Source: CAD feature listing. Evaluate the final solid. Frame: model axes, mm. A direction names the side the tool comes from. Give positions to 0.01 mm unless a question says otherwise; leave off trailing zeros. Order: outer loops, then holes, each group sorted by start corner. A loop starts at its lowest first (then second) coordinate and runs counter-clockwise, first axis right, second up.
```python
from build123d import *

# Parameters (mm, degrees)
SKETCH1_W               = 41
SKETCH1_H               = 30
BOSS_EXTRUDE1_DEPTH     = 20.4
SHELL1_T                = 2
BOSS_EXTRUDE2_START     = -2
BOSS_EXTRUDE2_OUTLINE_W = 5
BOSS_EXTRUDE2_OUTLINE_H = 20.4
BOSS_EXTRUDE2_OUTLINE_R = 2.25
BOSS_EXTRUDE2_DEPTH     = 2
SKETCH3_W               = 5
SKETCH3_H               = 2
BOSS_EXTRUDE3_DEPTH     = 2
SKETCH4_W               = 5
SKETCH4_H               = 2
BOSS_EXTRUDE4_DEPTH     = 2
SKETCH5_W               = 5
SKETCH5_H               = 2
BOSS_EXTRUDE5_DEPTH     = 2
SKETCH6_W               = 5
SKETCH6_H               = 2
BOSS_EXTRUDE6_DEPTH     = 2
SKETCH7_W               = 5
SKETCH7_H               = 30
BOSS_EXTRUDE7_DEPTH     = 1
SKETCH9_R               = 4.146052681
CUT_EXTRUDE4_DEPTH      = 11
SKETCH10_W              = 55
SKETCH10_H              = 32
BOSS_EXTRUDE9_DEPTH     = 2
BOSS_EXTRUDE10_DEPTH    = 3
FILLET1_R               = 1
SKETCH18_W              = 26.995153054
SKETCH18_H              = 16.789310936
CUT_EXTRUDE5_DEPTH      = 10
SKETCH20_R              = 2.5
CUT_EXTRUDE7_DEPTH      = 10


# Read off the part's stored shape, not the designer's step: Boss-Extrude2
with BuildPart() as part:
    # Sketch1 → Boss-Extrude1 (new body)
    with BuildSketch(Plane(origin=(0, 0, 0), x_dir=(1, 0, 0), z_dir=(0, 1, 0))):
        with Locations((20.5, 15)):
            Rectangle(SKETCH1_W, SKETCH1_H)
    extrude(amount=BOSS_EXTRUDE1_DEPTH)

    # Shell1
    shell1_openings = [part.faces().sort_by_distance(p)[0] for p in [
        (20.5, 10.2, 0),
    ]]
    offset(amount=SHELL1_T, openings=shell1_openings, kind=Kind.INTERSECTION)

    # Boss-Extrude2 outline → Boss-Extrude2 (add)
    # profile 1 of 2: a face of its own
    with BuildSketch(Plane.XY.offset(BOSS_EXTRUDE2_START)):
        with Locations((-4.5, 10.2)):
            Rectangle(BOSS_EXTRUDE2_OUTLINE_W, BOSS_EXTRUDE2_OUTLINE_H)
        with Locations((-4.5, 5.5)):
            Circle(BOSS_EXTRUDE2_OUTLINE_R, mode=Mode.SUBTRACT)
        with Locations((-4.5, 14.9)):
            Circle(BOSS_EXTRUDE2_OUTLINE_R, mode=Mode.SUBTRACT)
    # profile 2 of 2: a face of its own
    with BuildSketch(Plane.XY.offset(BOSS_EXTRUDE2_START)):
        with Locations((45.5, 10.2)):
            Rectangle(BOSS_EXTRUDE2_OUTLINE_W, BOSS_EXTRUDE2_OUTLINE_H)
        with Locations((45.5, 5.5)):
            Circle(BOSS_EXTRUDE2_OUTLINE_R, mode=Mode.SUBTRACT)
        with Locations((45.5, 14.9)):
            Circle(BOSS_EXTRUDE2_OUTLINE_R, mode=Mode.SUBTRACT)
    extrude(amount=BOSS_EXTRUDE2_DEPTH)

    # Sketch3 → Boss-Extrude3 (add)
    with BuildSketch(Plane(origin=(0, 20.4, 0), x_dir=(1, 0, 0), z_dir=(0, 1, 0))):
        with Locations((-4.5, 1)):
            Rectangle(SKETCH3_W, SKETCH3_H)
    extrude(amount=BOSS_EXTRUDE3_DEPTH)

    # Sketch4 → Boss-Extrude4 (add)
    with BuildSketch(Plane.XZ):
        with Locations((-4.5, -1)):
            Rectangle(SKETCH4_W, SKETCH4_H)
    extrude(amount=BOSS_EXTRUDE4_DEPTH)

    # Sketch5 → Boss-Extrude5 (add)
    with BuildSketch(Plane(origin=(0, 20.4, 0), x_dir=(1, 0, 0), z_dir=(0, 1, 0))):
        with Locations((45.5, 1)):
            Rectangle(SKETCH5_W, SKETCH5_H)
    extrude(amount=BOSS_EXTRUDE5_DEPTH)

    # Sketch6 → Boss-Extrude6 (add)
    with BuildSketch(Plane.XZ):
        with Locations((45.5, -1)):
            Rectangle(SKETCH6_W, SKETCH6_H)
    extrude(amount=BOSS_EXTRUDE6_DEPTH)

    # Sketch7 → Boss-Extrude7 (add)
    with BuildSketch(Plane.XZ.offset(2)):
        Polygon((-7, -2), (-2, -2), (-2, -32), (43, -32), (43, -2), (48, -2), (48, 0), (-7, 0), align=None)
        with Locations((-4.5, -17)):
            Rectangle(SKETCH7_W, SKETCH7_H)
        with Locations((45.5, -17)):
            Rectangle(SKETCH7_W, SKETCH7_H)
    extrude(amount=BOSS_EXTRUDE7_DEPTH)

    # Sketch9 → Cut-Extrude4 (cut)
    with BuildSketch(Plane(origin=(0, 0, -2), x_dir=(-1, 0, 0), z_dir=(0, 0, -1))):
        with Locations((4.5, 5.5)):
            Circle(SKETCH9_R)
        with Locations((4.5, 14.9)):
            Circle(SKETCH9_R)
    cut_extrude4 = extrude(amount=CUT_EXTRUDE4_DEPTH, mode=Mode.SUBTRACT)

    # Mirror1: Cut-Extrude4 across plane
    add(cut_extrude4.mirror(Plane(origin=(20.5, 0, 0), x_dir=(0, 0, 1), z_dir=(1, 0, 0))), mode=Mode.SUBTRACT)

    # Sketch10 → Boss-Extrude9 (add)
    with BuildSketch(Plane.XZ.offset(3)):
        with Locations((20.5, -16)):
            Rectangle(SKETCH10_W, SKETCH10_H)
    extrude(amount=BOSS_EXTRUDE9_DEPTH)

    # Sketch11 → Boss-Extrude10 (add)
    with BuildSketch(Plane.XZ.offset(5)):
        Polygon((48, 0), (-7, 0), (-17, 0), (-17, -32), (-7, -32), (48, -32), (58, -32), (58, 0), align=None)
    extrude(amount=BOSS_EXTRUDE10_DEPTH)

    # Fillet1
    fillet1_edges = [part.edges().sort_by_distance(p)[0] for p in [
        (43, -2, -17),
        (-7, -5, -16),
        (48, -5, -16),
        (-2, -2, -17),
    ]]
    fillet(fillet1_edges, radius=FILLET1_R)

    # Sketch18 → Cut-Extrude5 (cut)
    with BuildSketch(Plane(origin=(43, 0, 0), x_dir=(0, 0, -1), z_dir=(1, 0, 0))):
        with Locations((16.002935908, 10.000980191)):
            Rectangle(SKETCH18_W, SKETCH18_H)
    extrude(amount=-CUT_EXTRUDE5_DEPTH, mode=Mode.SUBTRACT)

    # Sketch20 → Cut-Extrude7 (cut)
    with BuildSketch(Plane(origin=(0, 0, 0), x_dir=(1, 0, 0), z_dir=(0, 1, 0))):
        with Locations(Location((-12.442315246, 16, 0), (0, 0, 270))):
            Circle(SKETCH20_R)
        with Locations(Location((53.442315246, 16, 0), (0, 0, 270))):
            Circle(SKETCH20_R)
    extrude(amount=-CUT_EXTRUDE7_DEPTH, mode=Mode.SUBTRACT)


solid = part.part
```
1) Section query D-D, the plane y = 19.5. Return the cut outline in (x, z).
Report:
outline: (-7, -2) - (-2, -2) - (-2, -32) - (43, -32) - (43, -2) - (48, -2) - (48, 0) - (41, 0) - (41, -30) - (0, -30) - (0, 0) - (-7, 0) - close
2) Draft query along Z for faces 5 (the flat face through (20, 22.4, -16)), 6 (the cylindrical face through (51, -6.48, -16.54)), 7 (the cylindrical face through (41.354, 5.554, -2.249)). Return one class per face: +Z half, -Z half, draft (parallel to the pull), parting line (faces both ways), or undercut.
Report:
face 5: draft
face 6: undercut
face 7: undercut
3) Reachability of faces 1 (the flat face through (42, 1.606, -16)), 2 (the cylindrical face through (-0.354, 14.954, -7.423)), 3 (the flat face through (48, -2.5, -9)), 4 (the flat face through (20, 0, -15)) from +Z, -Z, +X, -X, +Y, -Y: full face, straight path, thin tool, end or side. Return the list, or none.
Report:
face 1: +X
face 2: -X
face 3: +Z, -Z, +X, +Y
face 4: +Z
4) Section query B-B, the plane y = 14.9. Return the cut outline in (x, z).
Report:
outline: (-7, -2) - (-6.75, -2) - (-6.75, 0) - (-7, 0) - close; (-2.25, -2) - (-0.35, -2) - (-0.35, -13) - (-2, -13) - (-2, -32) - (43, -32) - (43, -29.5) - (41, -29.5) - (41, -30) - (0, -30) - (0, 0) - (-2.25, 0) - close; (41, -2.51) - (41.35, -2.51) - (41.35, -2) - (43.25, -2) - (43.25, 0) - (41, 0) - close; (47.75, -2) - (48, -2) - (48, 0) - (47.75, 0) - close
5) Pin query (flat end, axial travel): pin 1 (10 mm diameter, centred on y = 5.5, z = -14, fed in from -X); pin 2 (1.5 mm diameter, centred on x = -5, y = 8, fed in from -Z); pin 3 (1.2 mm diameter, centred on x = -5.5, z = -18.5, fed in from +Y); pin 4 (2.5 mm diameter, centred on x = -4.5, y = 14.9, fed in from +Z). Return the tip coordinate at first contact, or that it passes through.
Report:
pin 1: stops at x = -2
pin 2: stops at z = -2
pin 3: stops at y = -2
pin 4: passes through
6) Material intervals for L1, parallel to X at y = -6.85, z = -16; L2, parallel to Y at x = 1.5, z = -21; L3, parallel to Z at x = 10.5, y = 6.5, sorted ascending.
Report:
L1: x = -17 to -14.94, -9.94 to 50.94, 55.94 to 58
L2: y = -8 to 0, 20.4 to 22.4
L3: z = -32 to -30
7) Section query C-C, the plane x = 45.5. Return the cut outline in (y, z), and give its area (3 significant figures).
Report:
outline: (-8, -32) - (-2, -32) - (-2, -2) - (3.25, -2) - (3.25, 0) - (-8, 0) - close; (7.75, -2) - (12.65, -2) - (12.65, 0) - (7.75, 0) - close; (17.15, -2) - (22.4, -2) - (22.4, 0) - (17.15, 0) - close
area: 223 mm2
8) Section query A-A, the plane z = -16. Count the separate pieces of the cut face and the enclosed holes in it, and give its area (3 significant figures).
Report:
separate pieces: 3
enclosed holes: 0
area: 589 mm2
